Print and shaded views of the part. All mm, measured from the part's lowest x, y and z. A direction names the side the tool comes from. Round coordinates to 2 decimals unless told otherwise and drop trailing zeros. Order: outer loops, then holes, each group sorted by start corner. A loop starts at its lowest first (then second) coordinate and runs counter-clockwise, first axis right, second up. Notation, with made-up numbers: M 78,85.25 L 127,85.25 A26 ccw 127,118.25 Z; hole C 26,18 d8. An arc over 180 degrees is marked long. Write each question's results on one line, items separated by ' | '. Start each with the question number.
1. Band-saw the part on C-C, the plane y = 4.18. List the corners of the cut face in (x, z).
2. Drop flat-ended pins along their axis: pin 1 Ø3.5 at (x, y) = (54.5, 5.5) entering from -Z; pin 2 Ø6 at (x, y) = (8.5, 3.5) entering from -Z; pin 3 Ø1 at (x, y) = (19, 5) entering from +Z. Give the stop position or say it passes through.
3. Probe L1, parallel to X at y = 4.18, z = 3; L2, parallel to Y at x = 41.75, z = 3.75; L3, parallel to Z at x = 29.5, y = 6.5. List the from-to ranges inside material, lowest first. Write a range as [from, to].
4. Band-saw the part on D-D, the plane z = 10.5. List the corners of the cut face in (x, y), then the cut area to 3 significant figures.
5. Which spindle directions (+Z, -Z, +X, -X, +Y, -Y) get a long thin tool onto all of the face, cutting with end or side? Do the marked faces 1, 2 and 3. Say none if no direction does.
6. Band-saw the part on B-B, the plane x = 18.25. List the corners of the cut face in (y, z), then the cut area to 3 significant figures.
7. Band-saw the part on A-A, the plane z = 2.25. List the corners of the cut face in (x, y).
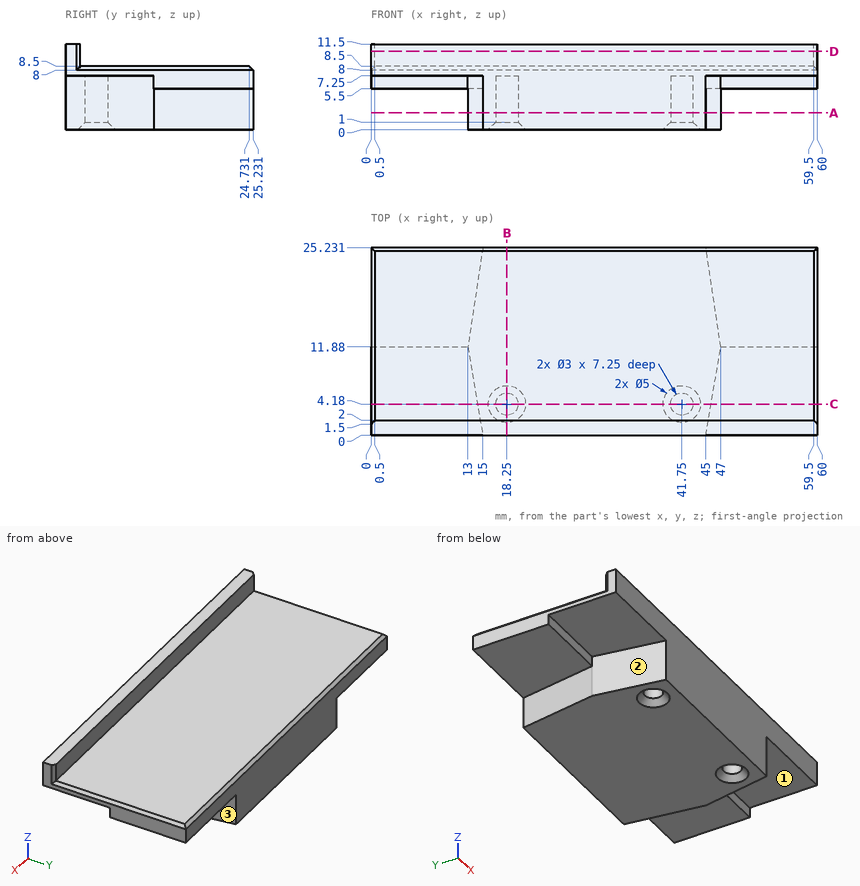
Solution:
1) outline: M 0,7.25 L 14.3,7.25 L 14.3,0 L 15.75,0 L 16.75,1 L 16.75,7.25 L 19.75,7.25 L 19.75,1 L 20.75,0 L 39.25,0 L 40.25,1 L 40.25,7.25 L 43.25,7.25 L 43.25,1 L 44.25,0 L 45.7,0 L 45.7,7.25 L 60,7.25 L 60,8 L 59.5,8.5 L 0.5,8.5 L 0,8 Z
2) pin 1: z = 7.25 | pin 2: z = 7.25 | pin 3: z = 8.5
3) L1: [14.3, 16.75], [19.75, 40.25], [43.25, 45.7] | L2: [0, 2.68], [5.68, 25.23] | L3: [0, 8.5]
4) outline: M 0,0 L 60,0 L 60,1.5 L 59.5,2 L 0.5,2 L 0,1.5 Z | area: 120 mm^2
5) face 1: -Z, +X, -Y | face 2: -Z, -X, -Y | face 3: -Z, +X, +Y
6) outline: M 0,0 L 1.68,0 L 2.68,1 L 2.68,7.25 L 5.68,7.25 L 5.68,1 L 6.68,0 L 25.23,0 L 25.23,8 L 24.73,8.5 L 2,8.5 L 2,11.5 L 0,11.5 Z | area: 198 mm^2
7) outline: M 13,11.88 L 15,0 L 45,0 L 47,11.88 L 45,25.23 L 15,25.23 Z; hole C 18.25,4.18 d3; hole C 41.75,4.18 d3
